Autodesk Inventor part; units mm, degrees
ref_plane "YZ Plane" through (0, 0, 0) normal (1, 0, 0) x (0, 1, 0)
ref_plane "XZ Plane" through (0, 0, 0) normal (0, 1, 0) x (-1, 0, 0)
ref_plane "XY Plane" through (0, 0, 0) normal (0, 0, 1) x (1, 0, 0)
sketch "Sketch1" plane through (0, 0, 0) normal (0, 0, 1) x (1, 0, 0)
  line L0 (0, 0) -> (38.1, 0)
  line L1 (38.1, 0) -> (38.1, 28.575)
  line L2 (38.1, 28.575) -> (0, 28.575)
  line L3 (0, 28.575) -> (0, 0)
  circle A0 centre (6.35, 22.225) radius 2.54
  circle A1 centre (19.05, 22.225) radius 2.54
  circle A2 centre (31.75, 22.225) radius 2.54
  dimension "d0" = 38.1
  dimension "d1" = 28.575
  dimension "d5" = 5.08
  dimension "d8" = 5.08
  dimension "d9" = 5.08
extrude "Extrusion1" add sketch "Sketch1" along normal blind 1.5875
properties part number "flatPoly3ForCNC"
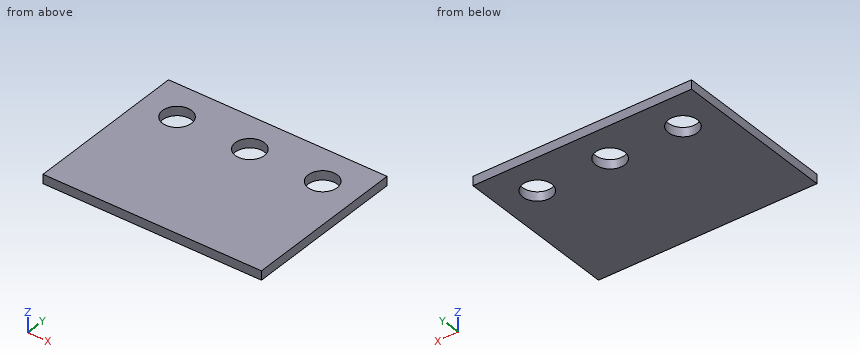
Design review of the part built by this model. Coordinates are the model's own, in mm. Round coordinates to 2 decimals unless told otherwise and drop trailing zeros. Order: outer loops, then holes, each group sorted by start corner. A loop starts at its lowest first (then second) coordinate and runs counter-clockwise, first axis right, second up. Notation, with made-up numbers: M 86.5,46.25 L 97.5,46.25 A19 cw 97.5,64.25 Z; hole C 30.5,31 d2. An arc over 180 degrees is marked long. Put each result on its own line as item: value.
Q1. Consider section A-A (x = 19.05). State the section outline as (y, z) points (1 decimal), and give its area (3 significant figures).
Reported:
outline: M 0,0 L 19.7,0 L 19.7,1.6 L 0,1.6 Z; M 24.8,0 L 28.6,0 L 28.6,1.6 L 24.8,1.6 Z
area: 37.3 mm²
Q2. Consider section D-D (x = 5). State the section outline as (y, z) points (1 decimal).
Reported:
outline: M 0,0 L 20.1,0 L 20.1,1.6 L 0,1.6 Z; M 24.4,0 L 28.6,0 L 28.6,1.6 L 24.4,1.6 Z
Q3. Consider section C-C (z = 0.25). State the section outline as (x, y) points (3 decimals).
Reported:
outline: M 0,0 L 38.1,0 L 38.1,28.575 L 0,28.575 Z; hole C 6.35,22.225 d5.08; hole C 19.05,22.225 d5.08; hole C 31.75,22.225 d5.08
Q4. Insertion check: pin 1 Ø2 at (x, y) = (12.5, 24) entering from -Z. The pin has a flat end and moves straight along its axis. Give the tip position at first contact, or say it passes through.
Reported:
pin 1: z = 0
Q5. Consider section B-B (y = 21.5). State the section outline as (x, z) points, and give its area (3 significant figures).
Reported:
outline: M 0,0 L 3.92,0 L 3.92,1.59 L 0,1.59 Z; M 8.78,0 L 16.62,0 L 16.62,1.59 L 8.78,1.59 Z; M 21.48,0 L 29.32,0 L 29.32,1.59 L 21.48,1.59 Z; M 34.18,0 L 38.1,0 L 38.1,1.59 L 34.18,1.59 Z
area: 37.3 mm²
Q6. To check wall thickness, follow line 1 (Y direction, x = 31.75, z = 1.2) (3 decimals); line 2 (Y direction, x = 34, z = 1.35) (3 decimals). State the ranges of each line that lie inside material, in increasing order.
Reported:
line 1: 0 to 19.685, 24.765 to 28.575
line 2: 0 to 21.046, 23.404 to 28.575
